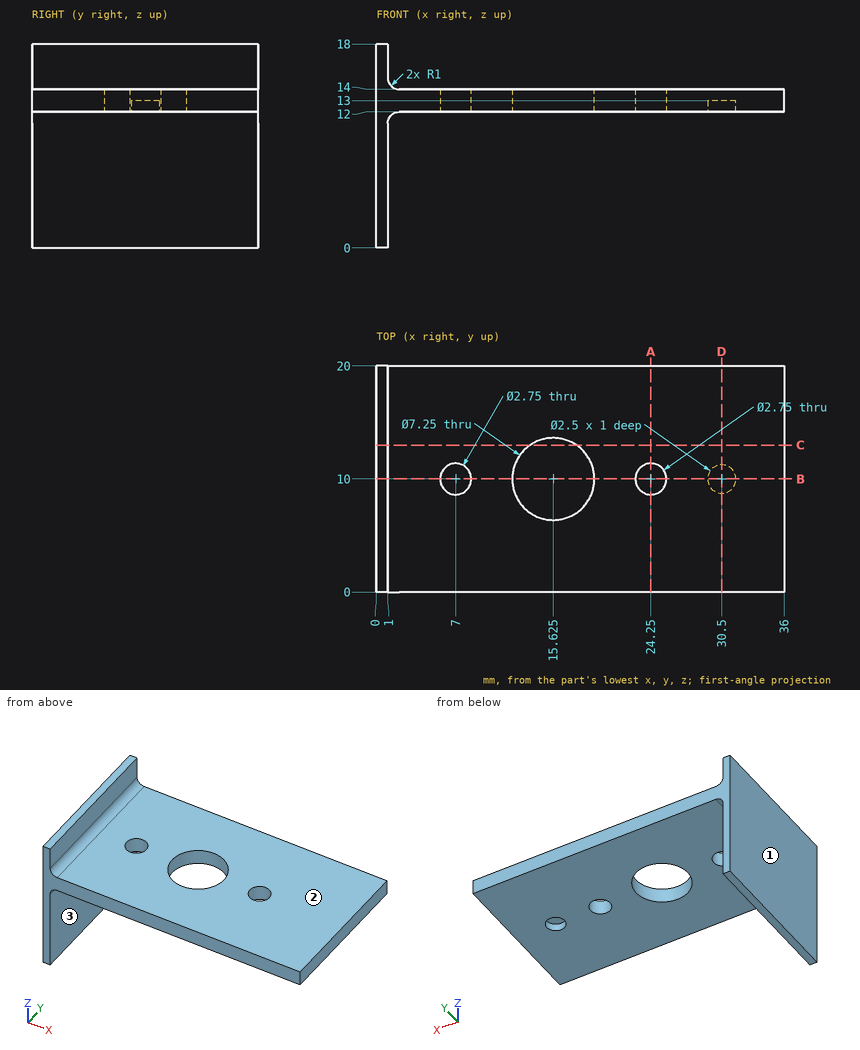
Print and shaded views of the part. All mm, measured from the part's lowest x, y and z. A direction names the side the tool comes from. Round coordinates to 2 decimals unless told otherwise and drop trailing zeros. Loops run counter-clockwise (first coordinate to the right, second up) from the corner with the lowest first, then second, coordinate; pieces in that order, holes last. Notation, with made-up numbers: (40, 26) -> (86, 26) arc R16 cw to (86, 57) -> close; hole circle Ø1 at (77, -40). An arc over 180 degrees is marked (long way). Use CSV: the item, a comma, the result in double quotes. Start each with the question number.
1) Drop flat-ended pins along their axis: P1, Ø3, axis at x = 30.5, y = 9.5, coming from the -Z side; P2, Ø2.5, axis at x = 7, y = 10, coming from the -Z side; P3, Ø1.5, axis at x = 30.5, y = 10, coming from the -Z side; P4, Ø1.5, axis at x = 12, y = 14.5, coming from the +Z side. Give the stop position or say it passes through.
2) Which spindle directions (+Z, -Z, +X, -X, +Y, -Y) get a long thin tool onto all of the face, cutting with end or side? Do the marked faces 1, 2 and 3. Say none if no direction does.
3) Wall check: L1, parallel to Y at x = 24.25, z = 12.5 (3 decimals); L2, parallel to Y at x = 30.5, z = 12.7; L3, parallel to X at y = 4.75, z = 2. Give the ranges that are in metal, low to high. Write a range as [from, to].
4) Cut at B-B, the plane y = 10. Write the cut outline in (x, z) (3 decimals).
5) Cut at D-D, the plane x = 30.5. Write the cut outline in (y, z).
6) Cut at C-C, the plane y = 13. Write the cut outline in (x, z).
7) Cut at A-A, the plane x = 24.25. Write the cut outline in (y, z) (3 decimals), plus the area to 3 significant figures.
Determined:
1,P1,"stops at z = 12"
1,P2,"passes through"
1,P3,"stops at z = 13"
1,P4,"stops at z = 14"
2,face 1,"+Z, -Z, -X, +Y, -Y"
2,face 2,"+Z, +X, +Y, -Y"
2,face 3,"-Z, +X, +Y, -Y"
3,L1,"y = [0, 8.625], [11.375, 20]"
3,L2,"y = [0, 8.75], [11.25, 20]"
3,L3,"x = [0, 1]"
4,outline,"(0, 0) -> (1, 0) -> (1, 11) arc R1 cw to (2, 12) -> (5.625, 12) -> (5.625, 14) -> (2, 14) arc R1 cw to (1, 15) -> (1, 18) -> (0, 18) -> close; (8.375, 12) -> (12, 12) -> (12, 14) -> (8.375, 14) -> close; (19.25, 12) -> (22.875, 12) -> (22.875, 14) -> (19.25, 14) -> close; (25.625, 12) -> (29.25, 12) -> (29.25, 13) -> (31.75, 13) -> (31.75, 12) -> (36, 12) -> (36, 14) -> (25.625, 14) -> close"
5,outline,"(0, 12) -> (8.75, 12) -> (8.75, 13) -> (11.25, 13) -> (11.25, 12) -> (20, 12) -> (20, 14) -> (0, 14) -> close"
6,outline,"(0, 0) -> (1, 0) -> (1, 11) arc R1 cw to (2, 12) -> (13.59, 12) -> (13.59, 14) -> (2, 14) arc R1 cw to (1, 15) -> (1, 18) -> (0, 18) -> close; (17.66, 12) -> (36, 12) -> (36, 14) -> (17.66, 14) -> close"
7,outline,"(0, 12) -> (8.625, 12) -> (8.625, 14) -> (0, 14) -> close; (11.375, 12) -> (20, 12) -> (20, 14) -> (11.375, 14) -> close"
7,area,"34.5 mm2"
